from build123d import *

# Parameters (mm, degrees)
SKETCH1_W           = 290
SKETCH1_H           = 195
BOSS_EXTRUDE1_DEPTH = 3
CUT_EXTRUDE1_DEPTH  = 10
SKETCH3_R           = 1.5
CUT_EXTRUDE2_DEPTH  = 10
CUT_EXTRUDE3_DEPTH  = 10
SKETCH5_W           = 20
SKETCH5_H           = 4.158505531
CUT_EXTRUDE4_DEPTH  = 10


with BuildPart() as part:
    # Sketch1 → Boss-Extrude1 (new body)
    with BuildSketch(Plane(origin=(0, 0, 0), x_dir=(0, 0, -1), z_dir=(1, 0, 0))):
        with Locations((-4.5, 3.341494469)):
            Rectangle(SKETCH1_W, SKETCH1_H)
    extrude(amount=BOSS_EXTRUDE1_DEPTH)

    # Sketch2 → Cut-Extrude1 (cut)
    with BuildSketch(Plane(origin=(3, 0, 0), x_dir=(0, 0, -1), z_dir=(1, 0, 0))):
        Polygon((-141.5, -94.158505531), (-141.5, -89.158505531), (-159.427644911, -89.158505531), (-159.427644911, -110.995569774), (-141.5, -110.995569774), align=None)
        Polygon((132.5, -110.995569774), (132.5, -94.158505531), (132.5, -89.158505531), (150.427644911, -89.158505531), (150.427644911, -110.995569774), align=None)
    extrude(amount=-CUT_EXTRUDE1_DEPTH, mode=Mode.SUBTRACT)

    # Sketch3 → Cut-Extrude2 (cut)
    with BuildSketch(Plane.ZY):
        with Locations((146.066251174, -64.158505531)):
            Circle(SKETCH3_R)
        with Locations((-137.061834429, -64.158505531)):
            Circle(SKETCH3_R)
        with Locations((-137.061834429, 5.841494469)):
            Circle(SKETCH3_R)
        with Locations((146.066251174, 5.841494469)):
            Circle(SKETCH3_R)
        with Locations((-137.061834429, 75.841494469)):
            Circle(SKETCH3_R)
        with Locations((146.066251174, 75.841494469)):
            Circle(SKETCH3_R)
        with Locations((-137.061834429, 90.841494469)):
            Circle(SKETCH3_R)
        with Locations((146.066251174, 90.841494469)):
            Circle(SKETCH3_R)
    extrude(amount=-CUT_EXTRUDE2_DEPTH, mode=Mode.SUBTRACT)

    # Sketch4 → Cut-Extrude3 (cut)
    with BuildSketch(Plane(origin=(3, 0, 0), x_dir=(0, 0, -1), z_dir=(1, 0, 0))):
        Polygon((-123.337688423, -74.726407598), (-90.571606652, -51.783350144), (-88.850877343, -54.240806276), (-121.616959114, -77.18386373), align=None)
        Polygon((-57.80552488, -28.84029269), (-25.039443109, -5.897235235), (-23.3187138, -8.354691368), (-56.084795571, -31.297748822), align=None)
        Polygon((7.726638663, 17.045822219), (40.492720435, 39.988879673), (42.213449744, 37.53142354), (9.447367972, 14.588366086), align=None)
    extrude(amount=-CUT_EXTRUDE3_DEPTH, mode=Mode.SUBTRACT)

    # Sketch5 → Cut-Extrude4 (cut)
    with BuildSketch(Plane(origin=(3, 0, 0), x_dir=(0, 0, -1), z_dir=(1, 0, 0))):
        with Locations((7.816456388, -2.079252766)):
            Rectangle(SKETCH5_W, SKETCH5_H)
        with Locations((47.816456388, -2.079252766)):
            Rectangle(SKETCH5_W, SKETCH5_H)
        with Locations((87.816456388, -2.079252766)):
            Rectangle(SKETCH5_W, SKETCH5_H)
    extrude(amount=-CUT_EXTRUDE4_DEPTH, mode=Mode.SUBTRACT)


solid = part.part
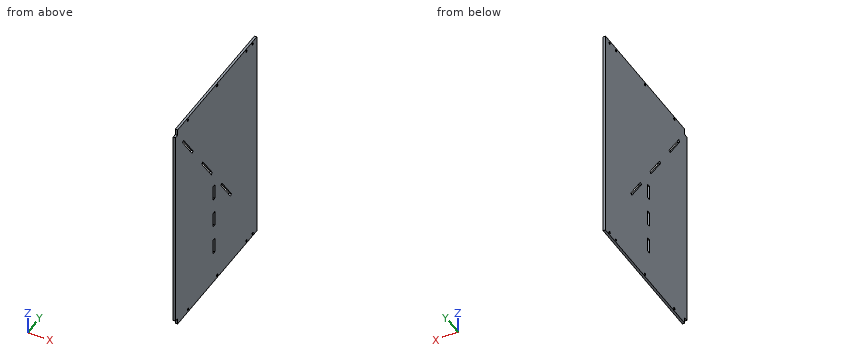
The listing builds one solid part. Answer for the finished solid, in the listing's coordinates (mm). Give positions to 0.01 mm unless a question says otherwise; leave off trailing zeros. Order: outer loops, then holes, each group sorted by start corner. A loop starts at its lowest first (then second) coordinate and runs counter-clockwise, first axis right, second up. Notation, with made-up numbers: (46, -6.75) -> (64, -6.75) arc R35 cw to (64, 26.25) -> close; hole circle Ø2 at (64, -33.75). An arc over 180 degrees is marked (long way). Put each result on its own line as item: value.
Item 1: Given P1, Ø0.9, axis at x = 1.5, z = 146.5, coming from the -Y side; P2, Ø1.5, axis at x = 2, y = -91.5, coming from the -Z side, each flat-ended and moving along its own axis, determine where each tip first touches the part or whether it passes through.
Established:
P1: stops at y = -89.16
P2: stops at z = -132.5
Item 2: A cutting plane is placed at A-A on z = -84. Give the vertices of the cut face in (x, y), plus the area to 3 significant figures.
Established:
outline: (0, -94.16) -> (3, -94.16) -> (3, -4.16) -> (0, -4.16) -> close; (0, 0) -> (3, 0) -> (3, 100.84) -> (0, 100.84) -> close
area: 573 mm^2
Item 3: A cutting plane is placed at B-B on y = 28.5. Give the vertices of the cut face in (x, z).
Established:
outline: (0, -140.5) -> (3, -140.5) -> (3, -29.32) -> (0, -29.32) -> close; (0, -24.08) -> (3, -24.08) -> (3, 149.5) -> (0, 149.5) -> close
Item 4: Straight lines are drawn through the part: line 1 (Z direction, x = 1.6, y = -2); line 2 (Z direction, x = 0.2, y = 91); line 3 (Y direction, x = 1.75, z = -87.5). For each, find the intervals that lie inside material, in ascending order.
Established:
line 1: z = -140.5 to -97.82, -77.82 to -57.82, -37.82 to -17.82, 2.18 to 149.5
line 2: z = -140.5 to -138.55, -135.57 to 144.57, 147.56 to 149.5
line 3: y = -94.16 to -4.16, 0 to 100.84
